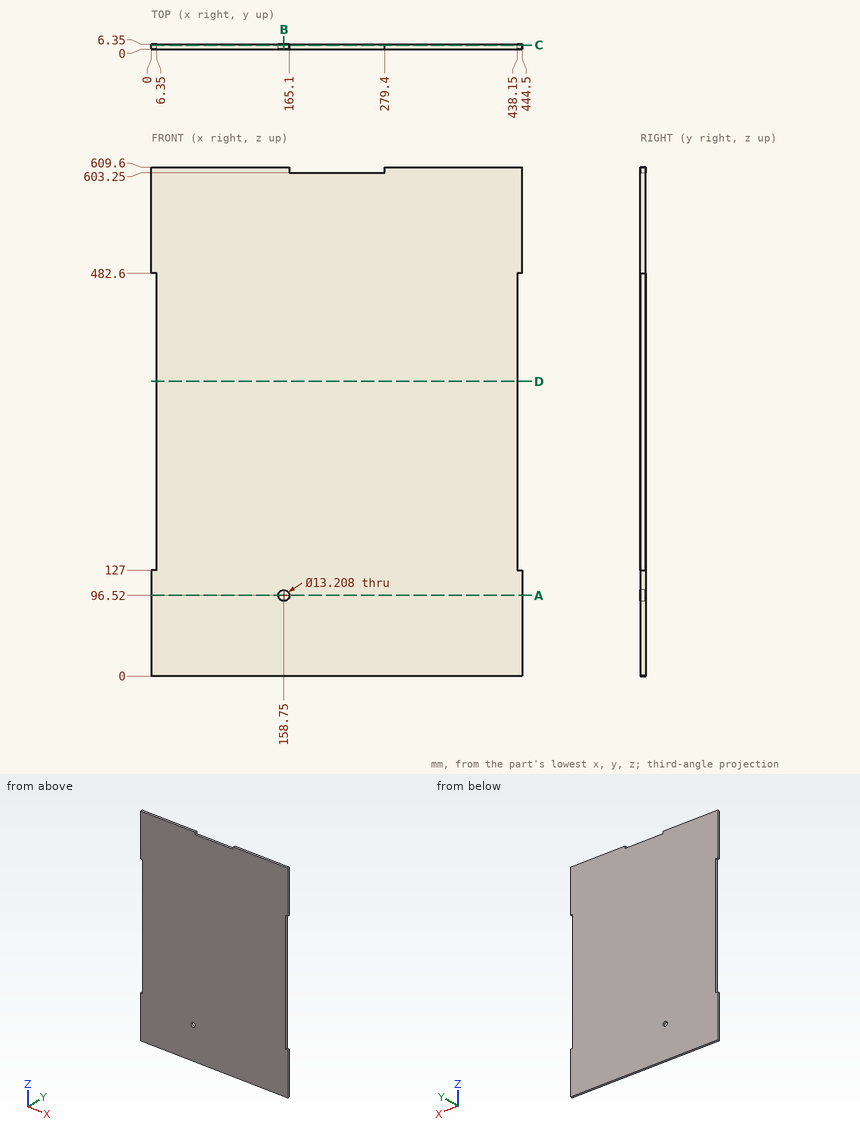
Verification items for this drawing (mm, ordinates from the low corner). Coordinates: 2 decimals unless noted, no trailing zeros. Order: outer loops, then holes, each group sorted by start corner. A loop starts at its lowest first (then second) coordinate and runs counter-clockwise, first axis right, second up. Notation, with made-up numbers: (-0.5, 54) - (37.5, 54) arc R20 cw to (37.5, 76) - close; hole circle Ø11 at (86.5, 3.5). An arc over 180 degrees is marked (long way). Answer in a Markdown table with one row per item. Add a question column.
1. Section check A-A (z = 96.52). Enter the section's corners in (x, y).
2. Section check D-D (z = 353). Enter the section's corners in (x, y), plus the area to 3 significant figures.
3. Section check B-B (x = 158.75). Enter the section's corners in (y, z), plus the area to 3 significant figures.
4. Material ranges on L1, parallel to Z at x = 158.75, y = 5.25; L2, parallel to X at y = 4, z = 96.52; L3, parallel to Z at x = 267, y = 0.5, recorded low to high. Write a range as [from, to].
5. Gauge pin test, flat ends, axial feed: pin 1 Ø8 at (x, z) = (158.75, 96.52) entering from -Y; pin 2 Ø1 at (y, z) = (1, 394) entering from +X; pin 3 Ø3 at (x, y) = (263.5, 5) entering from +Z. Record the tip position at first contact, or that the pin passes through.
6. Section check C-C (y = 5). Enter the section's corners in (x, z), plus the area to 3 significant figures.
Data:
| question | item | result |
|---|---|---|
| 1 | outline | (0, 0) - (152.15, 0) - (152.15, 6.35) - (0, 6.35) - close; (165.35, 0) - (444.5, 0) - (444.5, 6.35) - (165.35, 6.35) - close |
| 2 | outline | (6.35, 0) - (438.15, 0) - (438.15, 6.35) - (6.35, 6.35) - close |
| 2 | area | 2,740 mm² |
| 3 | outline | (0, 0) - (6.35, 0) - (6.35, 89.92) - (0, 89.92) - close; (0, 103.12) - (6.35, 103.12) - (6.35, 609.6) - (0, 609.6) - close |
| 3 | area | 3,790 mm² |
| 4 | L1 | z = [0, 89.92], [103.12, 609.6] |
| 4 | L2 | x = [0, 152.15], [165.35, 444.5] |
| 4 | L3 | z = [0, 603.25] |
| 5 | pin 1 | passes through |
| 5 | pin 2 | stops at x = 438.15 |
| 5 | pin 3 | stops at z = 603.25 |
| 6 | outline | (0, 0) - (444.5, 0) - (444.5, 127) - (438.15, 127) - (438.15, 482.6) - (444.5, 482.6) - (444.5, 609.6) - (279.4, 609.6) - (279.4, 603.25) - (165.1, 603.25) - (165.1, 609.6) - (0, 609.6) - (0, 482.6) - (6.35, 482.6) - (6.35, 127) - (0, 127) - close; hole circle Ø13.21 at (158.75, 96.52) |
| 6 | area | 266,000 mm² |
